from build123d import *

# Parameters (mm, degrees)
SKETCH1_W           = 8.89
SKETCH1_H           = 7.62
BOSS_EXTRUDE1_DEPTH = 25.4
SKETCH2_W           = 3.81
SKETCH2_H           = 17.78
CUT_EXTRUDE1_DEPTH  = 5.334
SKETCH3_W           = 2.54
SKETCH3_H           = 2.286
SKETCH3_H_2         = 2.54
BOSS_EXTRUDE2_DEPTH = 3.81
SKETCH4_W           = 3.81
SKETCH4_H           = 3.556
CUT_EXTRUDE2_DEPTH  = 3.286
SKETCH5_R           = 1.0414
CUT_EXTRUDE4_DEPTH  = 8.62
FILLET3_R           = 2.54
FILLET2_R           = 0.508


with BuildPart() as part:
    # Sketch1 → Boss-Extrude1 (new body)
    with BuildSketch(Plane(origin=(0, 0, 0), x_dir=(1, 0, 0), z_dir=(0, 1, 0))):
        Rectangle(SKETCH1_W, SKETCH1_H)
    extrude(amount=BOSS_EXTRUDE1_DEPTH)

    # Sketch2 → Cut-Extrude1 (cut)
    with BuildSketch(Plane.XY.offset(3.81)):
        with Locations((0, 12.7)):
            Rectangle(SKETCH2_W, SKETCH2_H)
    extrude(amount=-CUT_EXTRUDE1_DEPTH, mode=Mode.SUBTRACT)

    # Sketch3 → Boss-Extrude2 (add)
    with BuildSketch(Plane.ZY.offset(-1.905)):
        with Locations((-0.254, 14.351)):
            Rectangle(SKETCH3_W, SKETCH3_H)
        with Locations((-0.254, 8.509)):
            Rectangle(SKETCH3_W, SKETCH3_H)
        with Locations((-0.254, 20.32)):
            Rectangle(SKETCH3_W, SKETCH3_H_2)
    extrude(amount=BOSS_EXTRUDE2_DEPTH)

    # Sketch4 → Cut-Extrude2 (cut, through all)
    with BuildSketch(Plane.XY.offset(-1.524)):
        with Locations((0, 5.588)):
            Rectangle(SKETCH4_W, SKETCH4_H)
    extrude(amount=-CUT_EXTRUDE2_DEPTH, mode=Mode.SUBTRACT)

    # Sketch5 → Cut-Extrude4 (cut, through all)
    with BuildSketch(Plane.XY.offset(3.81)):
        with Locations((0, 2.032)):
            Circle(SKETCH5_R)
        with Locations((0, 23.368)):
            Circle(SKETCH5_R)
    extrude(amount=-CUT_EXTRUDE4_DEPTH, mode=Mode.SUBTRACT)

    # Fillet3
    fillet3_edges = [part.edges().sort_by_distance(p)[0] for p in [
        (-4.445, 25.4, 0),
        (4.445, 25.4, 0),
        (-4.445, 0, 0),
        (4.445, 0, 0),
    ]]
    fillet(fillet3_edges, radius=FILLET3_R)

    # Fillet2
    fillet2_edges = [part.edges().sort_by_distance(p)[0] for p in [
        (0, 25.4, -3.81),
        (4.445, 12.7, -3.81),
        (-3.701051224, 24.656051224, -3.81),
        (3.701051224, 24.656051224, -3.81),
        (3.701051224, 0.743948776, -3.81),
        (-3.701051224, 0.743948776, -3.81),
        (-4.445, 12.7, -3.81),
        (0, 0, -3.81),
    ]]
    fillet(fillet2_edges, radius=FILLET2_R)


solid = part.part
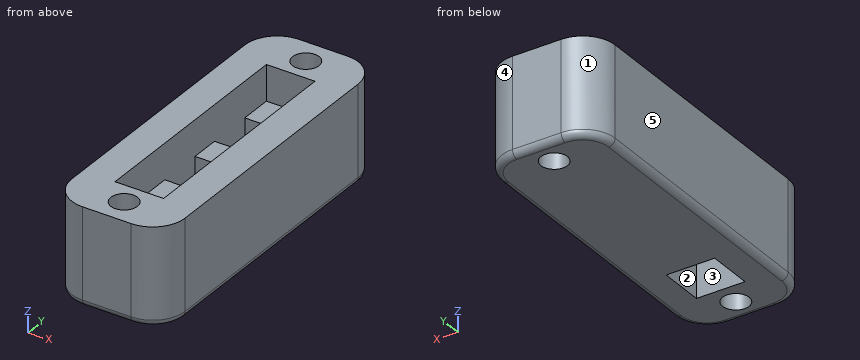
Here's how the part is built. I have some questions about the finished solid (model axes, mm). Face numbers are marked on the shaded views. A direction names the side the tool comes from. Give positions to 0.01 mm unless a question says otherwise; leave off trailing zeros. Order: outer loops, then holes, each group sorted by start corner. A loop starts at its lowest first (then second) coordinate and runs counter-clockwise, first axis right, second up. Notation, with made-up numbers: M 78,-10 L 104,-10 A33 cw 104,19 Z; hole C -23.5,58 d9. An arc over 180 degrees is marked long. Answer as a JSON object with one key per item and string values. Group by question number.
1) On a 3-axis mill with a long thin cutter (end or side, diameter ignored), from which of +Z, -Z, +X, -X, +Y, -Y can I reach the whole of each face in a straight line? I mean the marked faces 1 and 2. Say none if no direction works.
2) We'd pull the mould along X, two halves only. Please class the marked faces 3, 4 and 5: pulls with the +X half, pulls with the -X half, needs draft (parallel to the pull), parting line crosses it, or undercut.
3) Suppose I cut it at B-B, the plane y = 18. Write out the boundary of the cut face in (x, z) (3 decimals), plus the area to 3 significant figures.
4) Please list where these lines run through material, in increasing order: L1, parallel to Y at x = 0, z = -0.25; L2, parallel to Y at x = -1.75, z = 0.25; L3, parallel to Y at x = 0, z = 3.5. Write a range as [from, to].
5) I'm going to push a flat-ended pin straight in: pin 1 Ø0.7 at (x, y) = (0.5, 14.5) entering from +Z. Where does the tip first touch, or does it pass through?
6) Suppose I cut it at A-A, the plane x = 0. Write out the boundary of the cut face in (y, z).
7) Suppose I cut it at D-D, the plane z = 2.25. Write out the boundary of the cut face in (x, y) (3 decimals).
8) Suppose I cut it at C-C, the plane z = 0.75. Write out the boundary of the cut face in (x, y) (3 decimals), plus the area to 3 significant figures.
Results found:
{
 "1": {"face 1": "+Z, -Z, -X, +Y", "face 2": "+Z"},
 "2": {"face 3": "undercut", "face 4": "pulls with the +X half", "face 5": "pulls with the -X half"},
 "3": {"outline": "M -4.445,-3.302 A0.508 ccw -3.937,-3.81 L 3.937,-3.81 A0.508 ccw 4.445,-3.302 L 4.445,3.81 L 1.905,3.81 L 1.905,-1.524 L -1.905,-1.524 L -1.905,3.81 L -4.445,3.81 Z", "area": "47.3 mm²"},
 "4": {"L1": "[0, 0.99], [3.07, 3.81], [7.37, 9.65], [13.21, 15.49], [19.05, 22.33], [24.41, 25.4]", "L2": "[0, 3.81], [7.37, 9.65], [13.21, 15.49], [19.05, 25.4]", "L3": "[0, 0.99], [3.07, 3.81], [21.59, 22.33], [24.41, 25.4]"},
 "5": {"pin 1": "z = 1.02"},
 "6": {"outline": "M 0,-3.3 A0.51 ccw 0.51,-3.81 L 0.99,-3.81 L 0.99,3.81 L 0,3.81 Z; M 3.07,-3.81 L 3.81,-3.81 L 3.81,3.81 L 3.07,3.81 Z; M 7.37,-3.81 L 22.33,-3.81 L 22.33,3.81 L 21.59,3.81 L 21.59,1.02 L 19.05,1.02 L 19.05,-1.52 L 15.49,-1.52 L 15.49,1.02 L 13.21,1.02 L 13.21,-1.52 L 9.65,-1.52 L 9.65,1.02 L 7.37,1.02 Z; M 24.41,-3.81 L 24.89,-3.81 A0.51 ccw 25.4,-3.3 L 25.4,3.81 L 24.41,3.81 Z"},
 "7": {"outline": "M -4.445,2.54 A2.54 ccw -1.905,0 L 1.905,0 A2.54 ccw 4.445,2.54 L 4.445,22.86 A2.54 ccw 1.905,25.4 L -1.905,25.4 A2.54 ccw -4.445,22.86 Z; hole M -1.905,3.81 L 1.905,3.81 L 1.905,21.59 L -1.905,21.59 Z; hole C 0,2.032 d2.083; hole C 0,23.368 d2.083"},
 "8": {"outline": "M -4.445,2.54 A2.54 ccw -1.905,0 L 1.905,0 A2.54 ccw 4.445,2.54 L 4.445,22.86 A2.54 ccw 1.905,25.4 L -1.905,25.4 A2.54 ccw -4.445,22.86 Z; hole M -1.905,3.81 L 1.905,3.81 L 1.905,7.366 L -1.905,7.366 Z; hole M -1.905,9.652 L 1.905,9.652 L 1.905,13.208 L -1.905,13.208 Z; hole M -1.905,15.494 L 1.905,15.494 L 1.905,19.05 L -1.905,19.05 Z; hole C 0,2.032 d2.083; hole C 0,23.368 d2.083", "area": "173 mm²"}
}
